Geometry: final body of the model. Coordinates: model frame, mm. Round coordinates to 2 decimals unless told otherwise and drop trailing zeros. Use a Markdown table: item, result. Add a question column.
```python
from build123d import *

# Parameters (mm, degrees)
SKETCH1_W           = 431.8
SKETCH1_H           = 12.7
BOSS_EXTRUDE1_DEPTH = 0.381
SKETCH2_R           = 2.413
CUT_EXTRUDE1_DEPTH  = 1.381


with BuildPart() as part:
    # Sketch1 → Boss-Extrude1 (new body)
    with BuildSketch(Plane(origin=(0, 0, 0), x_dir=(1, 0, 0), z_dir=(0, 1, 0))):
        Rectangle(SKETCH1_W, SKETCH1_H)
    extrude(amount=BOSS_EXTRUDE1_DEPTH)

    # Sketch2 → Cut-Extrude1 (cut, through all)
    with BuildSketch(Plane(origin=(0, 0.381, 0), x_dir=(1, 0, 0), z_dir=(0, 1, 0))):
        Circle(SKETCH2_R)
        with Locations((-25.4, 0)):
            Circle(SKETCH2_R)
        with Locations((25.4, 0)):
            Circle(SKETCH2_R)
        with Locations((-50.8, 0)):
            Circle(SKETCH2_R)
        with Locations((-76.2, 0)):
            Circle(SKETCH2_R)
        with Locations((-101.6, 0)):
            Circle(SKETCH2_R)
        with Locations((-127, 0)):
            Circle(SKETCH2_R)
        with Locations((-152.4, 0)):
            Circle(SKETCH2_R)
        with Locations((-177.8, 0)):
            Circle(SKETCH2_R)
        with Locations((-203.2, 0)):
            Circle(SKETCH2_R)
        with Locations((50.8, 0)):
            Circle(SKETCH2_R)
        with Locations((76.2, 0)):
            Circle(SKETCH2_R)
        with Locations((101.6, 0)):
            Circle(SKETCH2_R)
        with Locations((127, 0)):
            Circle(SKETCH2_R)
        with Locations((152.4, 0)):
            Circle(SKETCH2_R)
        with Locations((177.8, 0)):
            Circle(SKETCH2_R)
        with Locations((203.2, 0)):
            Circle(SKETCH2_R)
    extrude(amount=-CUT_EXTRUDE1_DEPTH, mode=Mode.SUBTRACT)


solid = part.part
```
1) Section A-A, the plane y = 0.3. State how many separate pieces and enclosed holes the cut face has, then the cut area to 3 significant figures.
2) Pin query (flat end, axial travel): P1, Ø4.5, axis at x = -101.6, z = 0, coming from the -Y side. Return the tip coordinate at first contact, or that it passes through.
3) Material intervals for L1, parallel to Z at x = -101.6, y = 0.1, sorted ascending. Write a range as from..to.
Output values:
| question | item | result |
|---|---|---|
| 1 | separate pieces | 1 |
| 1 | enclosed holes | 17 |
| 1 | area | 5,170 mm^2 |
| 2 | P1 | passes through |
| 3 | L1 | z = -6.35..-2.41, 2.41..6.35 |
